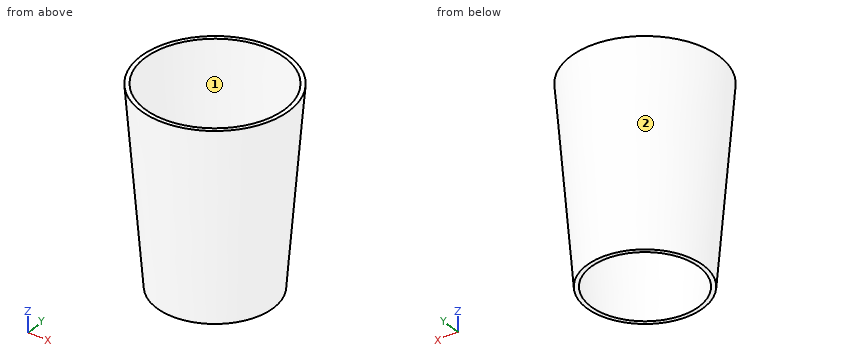
```python
from build123d import *


with BuildPart() as cone006:
    # Cone006 → Cone006 (revolve)
    with BuildSketch(Plane.XZ):
        Polygon((0, 0), (25.5, 0), (33, 92), (0, 92), align=None)
    revolve(axis=Axis((0, 0, 0), (0, 0, 1)))


with BuildPart() as cut006:
    # Cone005 → Cone005 (revolve)
    with BuildSketch(Plane.XZ):
        Polygon((0, 0), (27.5, 0), (35, 92), (0, 92), align=None)
    revolve(axis=Axis((0, 0, 0), (0, 0, 1)))

    # Cut006: cut Cone006
    add(cone006.part, mode=Mode.SUBTRACT)


solid = cut006.part
```
Can you work these out from the model? Positions are in its coordinate system, mm. Face numbers are marked on the shaded views. Coordinates: 2 decimals unless noted, no trailing zeros. Loops run counter-clockwise (first coordinate to the right, second up) from the corner with the lowest first, then second, coordinate; pieces in that order, holes last.
1) I need wall thicknesses on probe 1 along X at (y, z) = (4, 25); probe 2 along Y at (x, z) = (-23, 69); probe 3 along X at (y, z) = (-9, 80.5). Which ranges of each line are inside material? Lowest first, please.
2) Imagine slicing it at A-A on y = 0. List the corners of the cut face in (x, z) for me.
3) Imagine slicing it at C-C on z = 44. List the corners of the cut face in (x, y) for me, plus the area to 3 significant figures.
4) Imagine slicing it at D-D on z = 55. List the corners of the cut face in (x, y) for me.
5) Thinking about a two-plate mould opening in Y: for the marked faces 1 and 2, which applies, pulls with the +Y half, pulls with the -Y half, needs draft (parallel to the pull), parting line crosses it, or undercut?
6) For pin 1 (1 mm diameter, centred on x = -21.5, z = 58.5, fed in from +Y); pin 2 (1 mm diameter, centred on x = -3, z = 9.5, fed in from +Y); pin 3 (2 mm diameter, centred on y = 13, z = 64, fed in from -X), each with a flat end and sliding along its axis, tell me the tip position at first contact or that it passes through.
Completed:
1. probe 1: x = -29.27 to -27.25, 27.25 to 29.27
1. probe 2: y = -23.84 to -20.97, 20.97 to 23.84
1. probe 3: x = -32.85 to -30.77, 30.77 to 32.85
2. outline: (-35, 92) - (-27.5, 0) - (-25.5, 0) - (-33, 92) - close; (25.5, 0) - (27.5, 0) - (35, 92) - (33, 92) - close
3. outline: circle Ø62.17 at (0, 0); hole circle Ø58.17 at (0, 0)
3. area: 378 mm2
4. outline: circle Ø63.97 at (0, 0); hole circle Ø59.97 at (0, 0)
5. face 1: undercut
5. face 2: parting line crosses it
6. pin 1: stops at y = 24.5
6. pin 2: stops at y = 28.18
6. pin 3: stops at x = -30.45
